from build123d import *

# Parameters (mm, degrees)
SKETCH1_W           = 26.7
SKETCH1_H           = 26.7
BOSS_EXTRUDE1_DEPTH = 3.5
CHAMFER1_SIZE       = 2
SKETCH2_W           = 17
SKETCH2_H           = 16
BOSS_EXTRUDE2_DEPTH = 20
SKETCH3_W           = 9.899254973
SKETCH3_H           = 5.2
BOSS_EXTRUDE3_DEPTH = 20
SKETCH4_R           = 1.743878626
SKETCH4_W           = 2.182084489
SKETCH4_H           = 7.64251661
SKETCH4_W_2         = 2.305747791
SKETCH4_H_2         = 6.186643656
CUT_EXTRUDE1_DEPTH  = 5


with BuildPart() as part:
    # Sketch1 → Boss-Extrude1 (new body)
    with BuildSketch(Plane(origin=(0, 0, 0), x_dir=(1, 0, 0), z_dir=(0, 1, 0))):
        with Locations((-4.331476998, 13.35)):
            Rectangle(SKETCH1_W, SKETCH1_H)
    extrude(amount=BOSS_EXTRUDE1_DEPTH)

    # Chamfer1
    chamfer1_edges = [part.edges().sort_by_distance(p)[0] for p in [
        (9.018523002, 3.5, -13.35),
        (-4.331476998, 3.5, -26.7),
        (-17.681476998, 3.5, -13.35),
        (-4.331476998, 3.5, 0),
    ]]
    chamfer(chamfer1_edges, length=CHAMFER1_SIZE)

    # Sketch2 → Boss-Extrude2 (add)
    with BuildSketch(Plane.XZ):
        with Locations((-4.341476998, -11)):
            Rectangle(SKETCH2_W, SKETCH2_H)
    extrude(amount=BOSS_EXTRUDE2_DEPTH)

    # Sketch3 → Boss-Extrude3 (add)
    with BuildSketch(Plane.XZ):
        with Locations((-4.047830724, -21.6)):
            Rectangle(SKETCH3_W, SKETCH3_H)
    extrude(amount=BOSS_EXTRUDE3_DEPTH)

    # Sketch4 → Cut-Extrude1 (cut)
    with BuildSketch(Plane(origin=(0, 3.5, 0), x_dir=(1, 0, 0), z_dir=(0, 1, 0))):
        with Locations((-4.952893076, 19.999076914)):
            Circle(SKETCH4_R)
        with Locations((0.638087746, 9.527693342)):
            Rectangle(SKETCH4_W, SKETCH4_H)
        with Locations((-9.570218526, 9.483654221)):
            Rectangle(SKETCH4_W_2, SKETCH4_H_2)
    extrude(amount=-CUT_EXTRUDE1_DEPTH, mode=Mode.SUBTRACT)


solid = part.part
Input: part model. Units: mm. Frame: model coordinates. A direction names the side the tool comes from. Give positions to 0.01 mm unless a question says otherwise; leave off trailing zeros. Write each loop counter-clockwise with the first axis right and the second up, starting at its lowest first coordinate (ties: lowest second). Pieces come first, ordered by that corner, then holes. Notation, with made-up numbers: M 82,58.5 L 131,58.5 A22 cw 131,96.5 Z; hole C 41.25,-4.5 d8. An arc over 180 degrees is marked long. Write item = value, one per line. Start each with the question number.
1) Material intervals for line 1 along Z through (x, y) = (-10.75, -8); line 2 along X through (y, z) = (-18.25, -14.75); line 3 along Y through (x, z) = (7, -15), sorted ascending. Write a range as [from, to].
2) Cut plane A-A on y = -10.5. Return the cut outline in (x, z), then the cut area to 3 significant figures.
3) Cut plane C-C on x = -11.5. Return the cut outline in (y, z).
4) Cut plane D-D on y = 1. Return the cut outline in (x, z).
5) Reachability of faces 1 (the flat face through (9.019, 1, -13)), 2 (the flat face through (-12.841, -10, -11)), 3 (the flat face through (-0.453, 1, -9)), 4 (the flat face through (-8.997, -10, -22)), 5 (the flat face through (-4, 3.5, -14)) from +Z, -Z, +X, -X, +Y, -Y: full face, straight path, thin tool, end or side. Return the list, or none.
6) Cut plane B-B on z = -8. Return the cut outline in (x, y), then the cut area to 3 significant figures.
7) First-contact query: pin 1 Ø2 at (x, z) = (-14, -20) entering from -Y; pin 2 Ø3 at (x, z) = (-4.95, -20) entering from +Y; pin 3 Ø6 at (y, z) = (-16, -9) entering from +X. Flat tips, straight axial feed; report the tip coordinate or a pass-through.
8) Draft query along Z for faces 6 (the cylindrical face through (-5.331, 1.035, -18.297)), 7 (the flat face through (-4.5, 2.5, -1)), 8 (the flat face through (4.159, -10, -11)). Return one class per face: +Z half, -Z half, draft (parallel to the pull), parting line (faces both ways), or undercut.
Solved:
q1.line_1 = [-19, -3]
q1.line_2 = [-12.84, 4.16]
q1.line_3 = [0, 3.5]
q2.outline = M -12.84,-19 L -9,-19 L -9,-24.2 L 0.9,-24.2 L 0.9,-19 L 4.16,-19 L 4.16,-3 L -12.84,-3 Z
q2.area = 323 mm2
q3.outline = M -20,-19 L 0,-19 L 0,-26.7 L 1.5,-26.7 L 3.5,-24.7 L 3.5,-2 L 1.5,0 L 0,0 L 0,-3 L -20,-3 Z
q4.outline = M -17.68,-26.7 L 9.02,-26.7 L 9.02,0 L -17.68,0 Z; hole M -10.72,-12.58 L -8.42,-12.58 L -8.42,-6.39 L -10.72,-6.39 Z; hole C -4.95,-20 d3.49; hole M -0.45,-13.35 L 1.73,-13.35 L 1.73,-5.71 L -0.45,-5.71 Z
q5.face_1 = +Z, -Z, +X, +Y, -Y
q5.face_2 = +Z, -Z, -X, -Y
q5.face_3 = +Y
q5.face_4 = -Z, -X, -Y
q5.face_5 = +Z, -Z, +X, -X, +Y
q6.outline = M -17.68,0 L -12.84,0 L -12.84,-20 L 4.16,-20 L 4.16,0 L 9.02,0 L 9.02,1.5 L 7.02,3.5 L 1.73,3.5 L 1.73,-1.5 L -0.45,-1.5 L -0.45,3.5 L -8.42,3.5 L -8.42,-1.5 L -10.72,-1.5 L -10.72,3.5 L -15.68,3.5 L -17.68,1.5 Z
q6.area = 407 mm2
q7.pin_1 = 0
q7.pin_2 = -1.5
q7.pin_3 = 4.16
q8.face_6 = undercut
q8.face_7 = +Z half
q8.face_8 = draft
